Design review of the part built by this model. Coordinates are the model's own, in mm. Coordinates: 2 decimals unless noted, no trailing zeros. Write item = value, one per line.
```python
from build123d import *

# Parameters (mm, degrees)
SKETCH1_R               = 217
BOSS_EXTRUDE1_DEPTH     = 100
FILLET1_R               = 25
FILLET2_R               = 25
CUT_EXTRUDE4_DEPTH      = 20000
CUT_EXTRUDE4_DEPTH_BACK = 20000
CUT_EXTRUDE5_DEPTH      = 20000
CUT_EXTRUDE5_DEPTH_BACK = 20000
SKETCH8_R               = 25


with BuildPart() as part:
    # Sketch1 → Boss-Extrude1 (new body)
    with BuildSketch(Plane.XY):
        Circle(SKETCH1_R)
    extrude(amount=BOSS_EXTRUDE1_DEPTH)

    # Fillet1
    fillet1_edges = [part.edges().sort_by_distance(p)[0] for p in [
        (-217, 0, 100),
    ]]
    fillet(fillet1_edges, radius=FILLET1_R)

    # Fillet2
    fillet2_edges = [part.edges().sort_by_distance(p)[0] for p in [
        (-217, 0, 0),
    ]]
    fillet(fillet2_edges, radius=FILLET2_R)

    # Sketch3 → Cut-Extrude4 (cut, two sides: drawn at the far end of the back side and taken through both)
    with BuildSketch(Plane.XY.offset(-CUT_EXTRUDE4_DEPTH_BACK)):
        with BuildLine():
            ThreePointArc((-46, 0), (-45.116122899, -8.974154813), (-42.498458496, -17.603437889))
            Line((-42.498458496, -17.603437889), (-155.211761462, -64.290816637))
            ThreePointArc((-155.211761462, -64.290816637), (-164.771927108, -32.775174099), (-168, 0))
            Line((-168, 0), (-46, 0))
        make_face()
        with BuildLine():
            ThreePointArc((0, -46), (8.974154813, -45.116122899), (17.603437889, -42.498458496))
            Line((17.603437889, -42.498458496), (64.290816637, -155.211761462))
            ThreePointArc((64.290816637, -155.211761462), (32.775174099, -164.771927108), (0, -168))
            Line((0, -168), (0, -46))
        make_face()
        with BuildLine():
            ThreePointArc((32.526911935, -32.526911935), (38.247602166, -25.556230719), (42.498458496, -17.603437889))
            Line((42.498458496, -17.603437889), (155.211761462, -64.290816637))
            ThreePointArc((155.211761462, -64.290816637), (139.686894867, -93.335799147), (118.793939239, -118.793939239))
            Line((118.793939239, -118.793939239), (32.526911935, -32.526911935))
        make_face()
        with BuildLine():
            ThreePointArc((46, 0), (45.116122899, 8.974154813), (42.498458496, 17.603437889))
            Line((42.498458496, 17.603437889), (155.211761462, 64.290816637))
            ThreePointArc((155.211761462, 64.290816637), (164.771927108, 32.775174099), (168, 0))
            Line((168, 0), (46, 0))
        make_face()
        with BuildLine():
            ThreePointArc((32.526911935, 32.526911935), (25.556230719, 38.247602166), (17.603437889, 42.498458496))
            Line((17.603437889, 42.498458496), (64.290816637, 155.211761462))
            ThreePointArc((64.290816637, 155.211761462), (93.335799147, 139.686894867), (118.793939239, 118.793939239))
            Line((118.793939239, 118.793939239), (32.526911935, 32.526911935))
        make_face()
        with BuildLine():
            Line((0, 46), (0, 168))
            ThreePointArc((0, 168), (-32.775174099, 164.771927108), (-64.290816637, 155.211761462))
            Line((-64.290816637, 155.211761462), (-17.603437889, 42.498458496))
            ThreePointArc((-17.603437889, 42.498458496), (-8.974154813, 45.116122899), (0, 46))
        make_face()
        with BuildLine():
            Line((-42.498458496, 17.603437889), (-155.211761462, 64.290816637))
            ThreePointArc((-155.211761462, 64.290816637), (-139.686894867, 93.335799147), (-118.793939239, 118.793939239))
            Line((-118.793939239, 118.793939239), (-32.526911935, 32.526911935))
            ThreePointArc((-32.526911935, 32.526911935), (-38.247602166, 25.556230719), (-42.498458496, 17.603437889))
        make_face()
        with BuildLine():
            Line((-17.603437889, -42.498458496), (-64.290816637, -155.211761462))
            ThreePointArc((-64.290816637, -155.211761462), (-93.335799147, -139.686894867), (-118.793939239, -118.793939239))
            Line((-118.793939239, -118.793939239), (-32.526911935, -32.526911935))
            ThreePointArc((-32.526911935, -32.526911935), (-25.556230719, -38.247602166), (-17.603437889, -42.498458496))
        make_face()
    extrude(amount=CUT_EXTRUDE4_DEPTH + CUT_EXTRUDE4_DEPTH_BACK, mode=Mode.SUBTRACT)

    # Sketch8 → Cut-Extrude5 (cut, two sides: drawn at the far end of the back side and taken through both)
    with BuildSketch(Plane.XY.offset(-CUT_EXTRUDE5_DEPTH_BACK)):
        Circle(SKETCH8_R)
    extrude(amount=CUT_EXTRUDE5_DEPTH + CUT_EXTRUDE5_DEPTH_BACK, mode=Mode.SUBTRACT)


solid = part.part
```
(1) We need section A-A (z = 37.5). Give the number of separate pieces and of enclosed holes in the cut face, and give its area (3 significant figures).
Report:
separate_pieces = 1
enclosed_holes = 9
area = 105,000 mm²
(2) For L1, parallel to Y at x = -123, z = 24.5; L2, parallel to Y at x = -93, z = 76.5; L3, parallel to Y at x = 120.5, z = 26.5, list the stretches that pass through material, from the lowest coordinate up.
Report:
L1 = -178.77 to -50.95, 0 to 50.95, 114.43 to 178.77
L2 = -196.01 to -139.91, -93 to -38.52, 0 to 38.52, 93 to 196.01
L3 = -180.47 to -117.06, -49.91 to 0, 49.91 to 180.47
(3) Insertion check: pin 1 (1 mm diameter, centred on y = 152.5, z = 18.5, fed in from +X); pin 2 (8 mm diameter, centred on x = -112, y = 54, fed in from +Z); pin 3 (10 mm diameter, centred on y = -133.5, z = 61, fed in from +X); pin 4 (3 mm diameter, centred on x = -98.5, z = 46.5, fed in from -Y). Each pin has a flat end and moves straight along its axis. Give the tip position at first contact, or say it passes through.
Report:
pin_1 = 153.7
pin_2 = through
pin_3 = 174.86
pin_4 = -194.11
(4) The part is to be moulded in two halves that separate along X. For faces 1 (the cylindrical face through (206.98, 65.18, 49.65)), 2 (the cylindrical face through (33.23, -164.68, 49.3)), say which applies: released by +X, released by -X, zero draft, split by the parting line, or undercut.
Report:
face_1 = split by the parting line
face_2 = undercut
